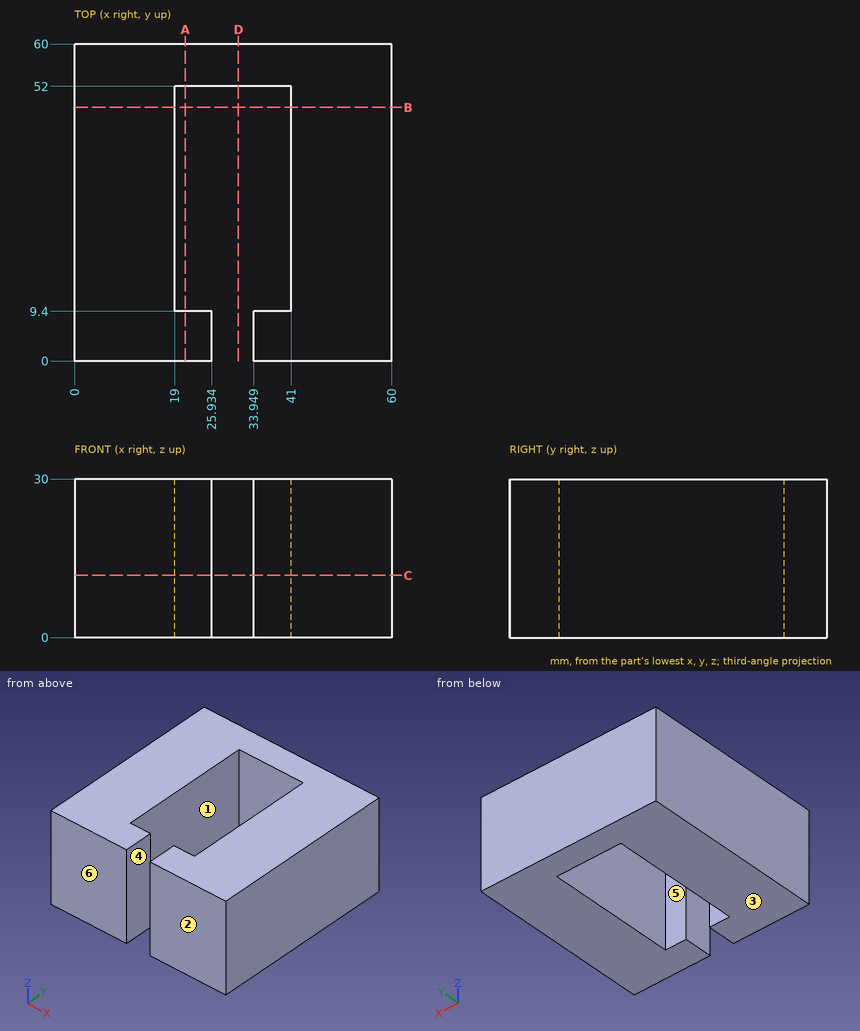
Design review of the part shown in the three views and the two pictorial views. Dimensions are in mm from the part's minimum x, y and z. A direction names the side the tool comes from. Round coordinates to 2 decimals unless told otherwise and drop trailing zeros. Loops run counter-clockwise (first coordinate to the right, second up) from the corner with the lowest first, then second, coordinate; pieces in that order, holes last. Notation, with made-up numbers: M -35.5,3.25 L 11.5,3.25 A21 ccw 11.5,32.25 Z; hole C 11,63 d10. An arc over 180 degrees is marked long. Write item = value, one per line.
Item 1: Take a section at A-A on x = 21. Write out the cut boundary in (y, z).
Return value:
outline = M 0,0 L 9.4,0 L 9.4,30 L 0,30 Z; M 52,0 L 60,0 L 60,30 L 52,30 Z
Item 2: Take a section at D-D on x = 31. Write out the cut boundary in (y, z).
Return value:
outline = M 52,0 L 60,0 L 60,30 L 52,30 Z
Item 3: Take a section at C-C on z = 11.75. Write out the cut boundary in (x, y), then the cut area to 3 significant figures.
Return value:
outline = M 0,0 L 25.93,0 L 25.93,9.4 L 19,9.4 L 19,52 L 41,52 L 41,9.4 L 33.95,9.4 L 33.95,0 L 60,0 L 60,60 L 0,60 Z
area = 2,590 mm2
Item 4: The part is to be moulded in two halves that separate along Y. For the marked faces 1, 2 and 3, say which applies: released by +Y, released by -Y, zero draft, split by the parting line, or undercut.
Return value:
face_1 = undercut
face_2 = released by -Y
face_3 = zero draft
Item 5: Machinability: for the marked faces 4, 5 and 6, which of the approach directions +Z, -Z, +X, -X, +Y, -Y give a long, thin tool a straight path to every point of the face, cutting with its end or side? Answer none if there is none.
Return value:
face_4 = +Z, -Z, -Y
face_5 = +Z, -Z
face_6 = +Z, -Z, +X, -X, -Y
Item 6: Take a section at B-B on y = 48. Write out the cut boundary in (x, z), then the cut area to 3 significant figures.
Return value:
outline = M 0,0 L 19,0 L 19,30 L 0,30 Z; M 41,0 L 60,0 L 60,30 L 41,30 Z
area = 1,140 mm2
Item 7: For line 1 (X direction, y = 29, z = 2.5); line 2 (Y direction, x = 34, z = 24); line 3 (X direction, y = 3, z = 22), list the stretches that pass through material, from the lowest coordinate up. Write a range as [from, to].
Return value:
line_1 = [0, 19], [41, 60]
line_2 = [0, 9.4], [52, 60]
line_3 = [0, 25.93], [33.95, 60]
